Source: three-view drawing plus pictorial views. Frame: mm from the lowest corner of the part. Give positions to 0.01 mm unless a question says otherwise; leave off trailing zeros. Order: outer loops, then holes, each group sorted by start corner. A loop starts at its lowest first (then second) coordinate and runs counter-clockwise, first axis right, second up. Notation, with made-up numbers: (-20.75, -25.5) - (33.25, -25.5) arc R26 ccw to (33.25, 3.5) - close; hole circle Ø7 at (17, -25). An arc over 180 degrees is marked (long way). Use one line per item in the form item = value.
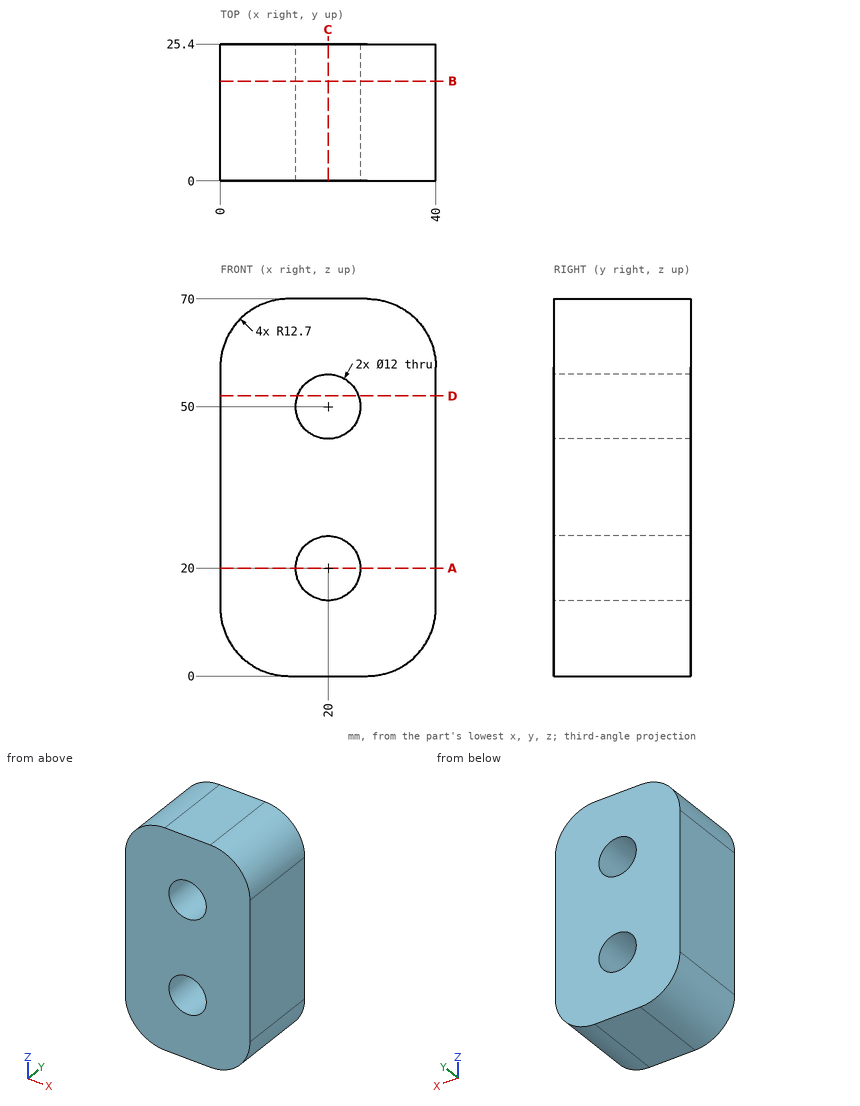
(1) Cut plane D-D on z = 52. Output: boundary loops of the cut face in (x, y).
Computed values:
outline = (0, 0) - (14.34, 0) - (14.34, 25.4) - (0, 25.4) - close; (25.66, 0) - (40, 0) - (40, 25.4) - (25.66, 25.4) - close
(2) Cut plane C-C on x = 20. Output: boundary loops of the cut face in (y, z), plus the area to 3 significant figures.
Computed values:
outline = (0, 0) - (25.4, 0) - (25.4, 14) - (0, 14) - close; (0, 26) - (25.4, 26) - (25.4, 44) - (0, 44) - close; (0, 56) - (25.4, 56) - (25.4, 70) - (0, 70) - close
area = 1,170 mm²
(3) Ray query, line 1 along Z through (x, y) = (20, 8.25); line 2 along Z through (x, y) = (22, 17.75); line 3 along X through (y, z) = (21.5, 22.5). Return the intervals inside material, ascending.
Computed values:
line_1 = 0 to 14, 26 to 44, 56 to 70
line_2 = 0 to 14.34, 25.66 to 44.34, 55.66 to 70
line_3 = 0 to 14.55, 25.45 to 40
(4) Cut plane B-B on y = 18.5. Output: boundary loops of the cut face in (x, z).
Computed values:
outline = (0, 12.7) arc R12.7 ccw to (12.7, 0) - (27.3, 0) arc R12.7 ccw to (40, 12.7) - (40, 57.3) arc R12.7 ccw to (27.3, 70) - (12.7, 70) arc R12.7 ccw to (0, 57.3) - close; hole circle Ø12 at (20, 20); hole circle Ø12 at (20, 50)
(5) Contact query for flat-ended pins moving along their axis: pin 1 Ø11 at (x, z) = (20, 20) entering from +Y; pin 2 Ø3 at (y, z) = (13, 62.5) entering from +X; pin 3 Ø3 at (y, z) = (15, 11) entering from -X; pin 4 Ø10 at (x, y) = (35, 12.5) entering from +Z. Output: stop coordinate, or through.
Computed values:
pin_1 = through
pin_2 = 39.45
pin_3 = 0
pin_4 = 69.71
(6) Cut plane A-A on z = 20. Output: boundary loops of the cut face in (x, y).
Computed values:
outline = (0, 0) - (14, 0) - (14, 25.4) - (0, 25.4) - close; (26, 0) - (40, 0) - (40, 25.4) - (26, 25.4) - close
